Geometry check sheet. Reference: the model listing, model coordinates, mm. Face numbers are marked on the shaded views. Coordinates: 2 decimals unless noted, no trailing zeros. Order: outer loops, then holes, each group sorted by start corner. A loop starts at its lowest first (then second) coordinate and runs counter-clockwise, first axis right, second up. Notation, with made-up numbers: M 79.25,20.5 L 113.25,20.5 A11 cw 113.25,24.5 Z; hole C -20.5,-24.75 d5. An arc over 180 degrees is marked long. One line per item, written item: value. Start each with the question number.
1) Go/stop test with flat-tipped pins: P1, Ø8, axis at y = 812, z = -167, coming from the -X side; P2, Ø8, axis at x = 490, z = -271.5, coming from the +Y side; P3, Ø5, axis at x = 341, y = 869.5, coming from the +Z side; P4, Ø12, axis at x = 164.5, z = -355.5, coming from the -Y side. Record where each tip stops, or that it passes through.
2) Draft check along X on the marked faces 1, 2, 3 and 4. Enter one of: pulls with the +X half, pulls with the -X half, needs draft (parallel to the pull), parting line crosses it, or undercut.
3) Sectioned sample at A-A, the plane y = 731. Enter the section's corners in (x, z).
4) Thickness scan on L1, parallel to Y at x = 543.5, z = -49; L2, parallel to Z at x = 426.5, y = 915; L3, parallel to Z at x = 62.5, y = 946. Record the ranges inside material, lowest first. Write a range as from..to.
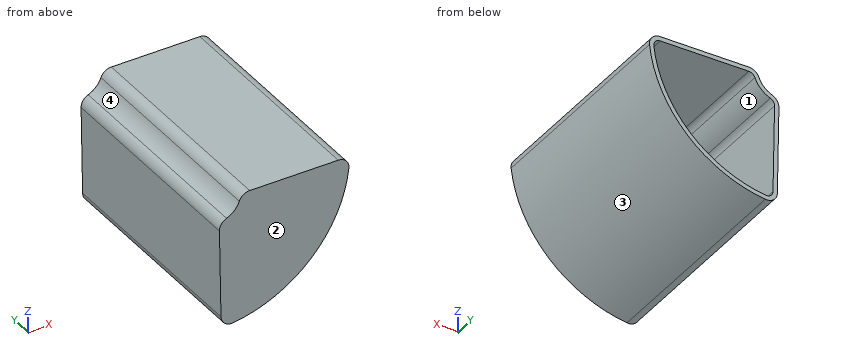
Autodesk Inventor part; units mm, degrees
ref_plane "YZ Plane" through (0, 0, 0) normal (1, 0, 0) x (0, 1, 0)
ref_plane "XZ Plane" through (0, 0, 0) normal (0, 1, 0) x (-1, 0, 0)
ref_plane "XY Plane" through (0, 0, 0) normal (0, 0, 1) x (1, 0, 0)
sketch "草图1" plane through (0, 0, 0) normal (0, 1, 0) x (-1, 0, 0)
  circle A0 centre (0, 0) radius 650
  arc A1 (-64.9652, -596.4726) -> (-9.5591, -547.6391) centre (-59.5515, -546.7665) ccw
  line L0 (-2.4681, -141.3998) -> (-9.5591, -547.6391)
  arc A2 (-2.4681, -141.3998) -> (-34.9737, -93.6848) centre (-52.4605, -140.5272) ccw
  arc A3 (-93.6848, -34.9737) -> (-34.9737, -93.6848) centre (0, 0) ccw
  arc A4 (-93.6848, -34.9737) -> (-141.3998, -2.4681) centre (-140.5272, -52.4605) ccw
  line L1 (-547.6391, -9.5591) -> (-141.3998, -2.4681)
  arc A5 (-547.6391, -9.5591) -> (-596.4726, -64.9652) centre (-546.7665, -59.5515) ccw
  arc A6 (-596.4726, -64.9652) -> (-64.9652, -596.4726) centre (0, 0) ccw
  arc A7 (-64.9652, -596.4726) -> (-9.5591, -547.6391) centre (-59.5515, -546.7665) ccw
  line L2 (-9.5591, -547.6391) -> (-2.4681, -141.3998)
  arc A8 (-2.4681, -141.3998) -> (-34.9737, -93.6848) centre (-52.4605, -140.5272) ccw
  arc A9 (-93.6848, -34.9737) -> (-34.9737, -93.6848) centre (0, 0) ccw
  arc A10 (-93.6848, -34.9737) -> (-141.3998, -2.4681) centre (-140.5272, -52.4605) ccw
  line L3 (-141.3998, -2.4681) -> (-547.6391, -9.5591)
  arc A11 (-547.6391, -9.5591) -> (-596.4726, -64.9652) centre (-546.7665, -59.5515) ccw
  arc A12 (-596.4726, -64.9652) -> (-64.9652, -596.4726) centre (0, 0) ccw
  line L4 (-22.4651, -141.0508) -> (-29.556, -547.2901)
  arc A13 (-62.7997, -576.5901) -> (-29.556, -547.2901) centre (-59.5515, -546.7665) ccw
  arc A14 (-576.5901, -62.7997) -> (-62.7997, -576.5901) centre (0, 0) ccw
  arc A15 (-547.2901, -29.556) -> (-576.5901, -62.7997) centre (-546.7665, -59.5515) ccw
  line L5 (-547.2901, -29.556) -> (-141.0508, -22.4651)
  arc A16 (-112.4218, -41.9684) -> (-141.0508, -22.4651) centre (-140.5272, -52.4605) ccw
  arc A17 (-112.4218, -41.9684) -> (-41.9684, -112.4218) centre (0, 0) ccw
  arc A18 (-22.4651, -141.0508) -> (-41.9684, -112.4218) centre (-52.4605, -140.5272) ccw
  dimension "d0" = 1300
  dimension "d3" = 0
  dimension "d4" = 20
extrude "拉伸2" add sketch "草图1" along normal blind 1000 contours A6 A5 L1 A4 A3 A2 L0 A1
extrude "拉伸3" add sketch "草图1" along normal blind 30 contours L4 A13 A14 A15 L5 A16 A17 A18
fillet "圆角1" radius 10 8 edges at (569.2726, 30, -39.7152) (344.1704, 30, -26.0106) (123.6368, 30, -27.6671) (84.8528, 30, -84.8528) (27.6671, 30, -123.6368) (26.0106, 30, -344.1704) (39.7152, 30, -569.2726) (410.1219, 30, -410.1219)
properties part number "桶"
Final values:
1. P1: stops at x = 2.85
1. P2: stops at y = 30
1. P3: stops at z = -5.91
1. P4: stops at y = 0
2. face 1: undercut
2. face 2: needs draft
2. face 3: pulls with the +X half
2. face 4: pulls with the -X half
3. outline: M 2.47,-141.4 L 9.56,-547.64 A50 ccw 64.97,-596.47 A600 ccw 596.47,-64.97 A50 ccw 547.64,-9.56 L 141.4,-2.47 A50 ccw 93.68,-34.97 A100 cw 34.97,-93.68 A50 ccw Z; hole M 22.47,-141.05 L 29.56,-547.29 A30 ccw 62.8,-576.59 A580 ccw 576.59,-62.8 A30 ccw 547.29,-29.56 L 141.05,-22.47 A30 ccw 112.42,-41.97 A120 cw 41.97,-112.42 A30 ccw Z
4. L1: y = 0..30
4. L2: z = -422.02..-393.06, -27.45..-7.44
4. L3: z = -596.68..-576.62, -102.44..-78.06
